Geometry check sheet. Reference: drawing and pictorial views, mm from the part's lowest x, y, z. Coordinates: 2 decimals unless noted, no trailing zeros. Loops run counter-clockwise (first coordinate to the right, second up) from the corner with the lowest first, then second, coordinate; pieces in that order, holes last. Notation, with made-up numbers: (26, 52.25) -> (81, 52.25) arc R23 cw to (81, 84.25) -> close; hole circle Ø9 at (29.25, -38.75). An arc over 180 degrees is marked (long way). Use one line per item in the form item = value.
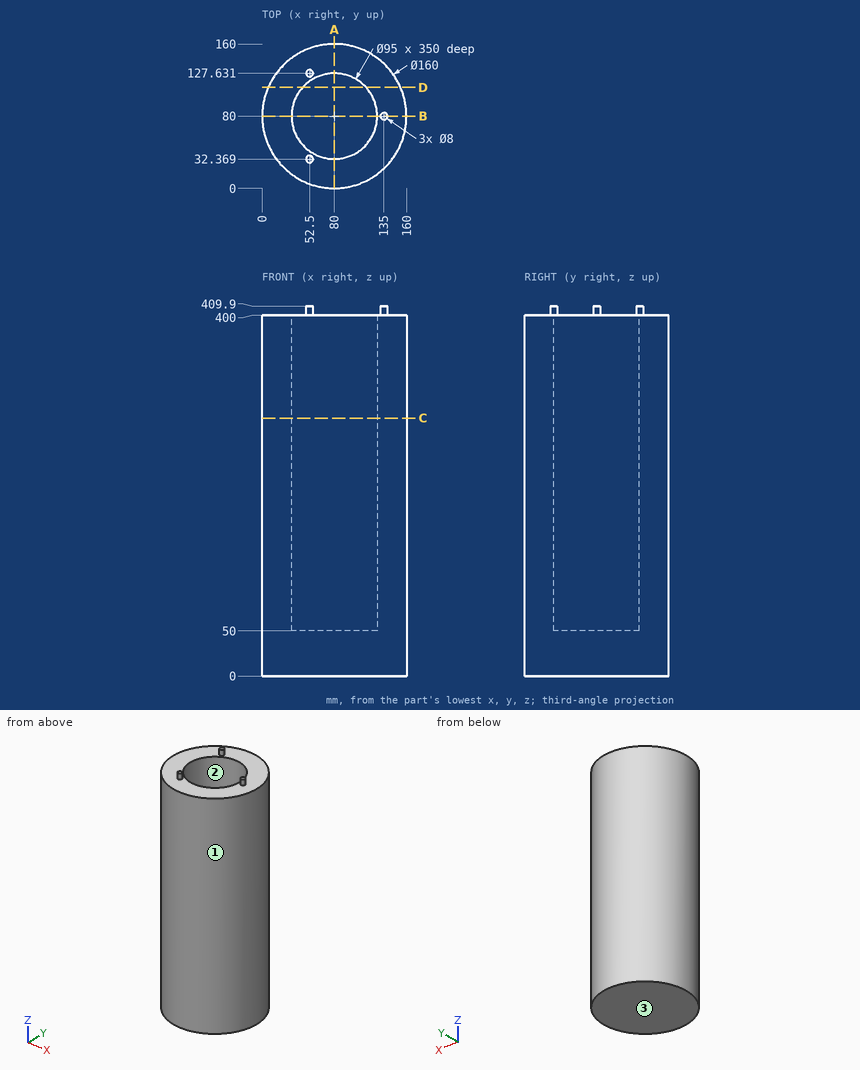
(1) Go/stop test with flat-tipped pins: P1, Ø12, axis at x = 87.5, z = 286, coming from the -Y side; P2, Ø2, axis at x = 107, z = 81.5, coming from the -Y side; P3, Ø6, axis at x = 34, y = 111, coming from the +Z side. Record where each tip stops, or that it passes through.
Established:
P1 = 0.01
P2 = 4.34
P3 = 400
(2) Section check C-C, the plane z = 286. Record the boundary of the cut face in (x, y), plus the area to 3 significant figures.
Established:
outline = circle Ø160 at (80, 80); hole circle Ø95 at (80, 80)
area = 13,000 mm²
(3) Mould release check, pull along X, two halves, no side actions. Record for the marked faces 1, 2 and 3: +X half, -X half, draft (parallel to the pull), parting line (faces both ways), or undercut.
Established:
face_1 = parting line
face_2 = undercut
face_3 = draft
(4) Scan lines: line 1 along Y through (x, z) = (80, 138.5); line 2 along Z through (x, y) = (115.5, 112.5); line 3 along Z through (x, y) = (102.5, 81). Record each from-to range of solid material in increasing order.
Established:
line_1 = 0 to 32.5, 127.5 to 160
line_2 = 0 to 400
line_3 = 0 to 50
(5) Section check A-A, the plane x = 80. Record the boundary of the cut face in (y, z), plus the area to 4 significant figures.
Established:
outline = (0, 0) -> (160, 0) -> (160, 400) -> (127.5, 400) -> (127.5, 50) -> (32.5, 50) -> (32.5, 400) -> (0, 400) -> close
area = 30,750 mm²
(6) Section check B-B, the plane y = 80. Record the boundary of the cut face in (x, z).
Established:
outline = (0, 0) -> (160, 0) -> (160, 400) -> (139, 400) -> (139, 409.9) -> (131, 409.9) -> (131, 400) -> (127.5, 400) -> (127.5, 50) -> (32.5, 50) -> (32.5, 400) -> (0, 400) -> close
(7) Section check D-D, the plane y = 112. Record the boundary of the cut face in (x, z).
Established:
outline = (6.68, 0) -> (153.32, 0) -> (153.32, 400) -> (115.1, 400) -> (115.1, 50) -> (44.9, 50) -> (44.9, 400) -> (6.68, 400) -> close
